Source: CAD feature listing. Evaluate the final solid. Frame: model axes, mm. A direction names the side the tool comes from. Give positions to 0.01 mm unless a question says otherwise; leave off trailing zeros. Write each loop counter-clockwise with the first axis right and the second up, starting at its lowest first coordinate (ties: lowest second). Pieces come first, ordered by that corner, then holes. Notation, with made-up numbers: M 33.25,37 L 39.25,37 A21 cw 39.25,72 Z; hole C 79.5,33 d4. An arc over 180 degrees is marked long. Return JSON: item names as keys, results as strings.
Autodesk Inventor part; units mm, degrees
ref_plane "YZ Plane" through (0, 0, 0) normal (1, 0, 0) x (0, 1, 0)
ref_plane "XZ Plane" through (0, 0, 0) normal (0, 1, 0) x (-1, 0, 0)
ref_plane "XY Plane" through (0, 0, 0) normal (0, 0, 1) x (1, 0, 0)
sketch "Sketch1" plane through (0, 0, 0) normal (0, 0, 1) x (1, 0, 0)
  line L0 (-0.7879, 4.5) -> (3.5032, 2.9324)
  line L1 (3.5032, 2.9324) -> (4.2911, -1.5676)
  line L2 (4.2911, -1.5676) -> (0.7879, -4.5)
  line L3 (0.7879, -4.5) -> (-3.5032, -2.9324)
  line L4 (-3.5032, -2.9324) -> (-4.2911, 1.5676)
  line L5 (-4.2911, 1.5676) -> (-0.7879, 4.5)
  point P0 (0, 0)
  point P1 (0, 0)
  dimension "d0" = 9
extrude "Extrusion1" add sketch "Sketch1" along normal blind 3
sketch "Sketch2" plane through (0, 0, 3) normal (0, 0, 1) x (1, 0, 0)
  circle A0 centre (0, 0) radius 3
  dimension "d3" = 6
extrude "Extrusion2" add sketch "Sketch2" along normal blind 1
sketch "Sketch3" plane through (0, 0, 4) normal (0, 0, 1) x (1, 0, 0)
  line L0 (-0.7879, 4.5) -> (-4.2911, 1.5676)
  line L1 (-0.7879, 4.5) -> (3.5032, 2.9324)
  line L2 (3.5032, 2.9324) -> (4.2911, -1.5676)
  line L3 (4.2911, -1.5676) -> (0.7879, -4.5)
  line L4 (0.7879, -4.5) -> (-3.5032, -2.9324)
  line L5 (-3.5032, -2.9324) -> (-4.2911, 1.5676)
  line L6 (-4.2911, 1.5676) -> (-0.7879, 4.5)
  point P0 (0, 0)
  point P1 (0, 0)
extrude "Extrusion3" add sketch "Sketch3" along normal blind 3
sketch "Sketch4" plane through (0, 0, 7) normal (0, 0, 1) x (1, 0, 0)
  circle A0 centre (0, 0) radius 3
  dimension "d8" = 6
extrude "Extrusion4" add sketch "Sketch4" along normal blind 22
thread "Thread1"
properties part number "HUDOSN-1-54B"
1) Set-up query: faces 4 (the face through (-3, 0, 18)), 5 (the face through (-3, -0.1, 3.5)), 6 (the face through (-1.328, -3.727, 1.479)). Return all of +Z, -Z, +X, -X, +Y, -Y with unobstructed straight access to the full face (end or side cutting, diameter ignored); none if empty.
Numbers:
{"face 4": "+Z", "face 5": "none", "face 6": "+Z, -Z, -X, -Y"}
2) Cut plane A-A, the plane y = 3.75. Return the cut outline in (x, z), then the cut area to 3 significant figures.
Numbers:
{"outline": "M -1.68,0 L 1.27,0 L 1.27,3 L -1.68,3 Z; M -1.68,4 L 1.27,4 L 1.27,7 L -1.68,7 Z", "area": "17.7 mm²"}
3) Contact query for flat-ended pins moving along their axis: pin 1 Ø5 at (x, z) = (1, 23.5) entering from -Y; pin 2 Ø1 at (y, z) = (1.5, 16) entering from -X; pin 3 Ø1.5 at (y, z) = (3, 16.5) entering from +X. Output: stop coordinate, or through.
Numbers:
{"pin 1": "stops at y = -3", "pin 2": "stops at x = -2.83", "pin 3": "stops at x = 1.98"}
4) Cut plane C-C, the plane z = 11.25. Return the cut outline in (x, y), then the cut area to 3 significant figures.
Numbers:
{"outline": "C 0,0 d6", "area": "28.3 mm²"}
5) Cut plane B-B, the plane x = -0.5. Return the cut outline in (y, z).
Numbers:
{"outline": "M -4.03,0 L 4.39,0 L 4.39,3 L 2.96,3 L 2.96,4 L 4.39,4 L 4.39,7 L 2.96,7 L 2.96,29 L -2.96,29 L -2.96,7 L -4.03,7 L -4.03,4 L -2.96,4 L -2.96,3 L -4.03,3 Z"}
6) Draft query along Z for faces 1 (the face through (-1, -3, 7)), 2 (the face through (-1, -3, 3)), 3 (the face through (2.564, -3.013, 1.479)). Return one class per face: released by +Z, released by -Z, zero draft, split by the parting line, or undercut.
Numbers:
{"face 1": "released by +Z", "face 2": "undercut", "face 3": "zero draft"}
7) Line query: line 1 (Z direction, x = 3.75, y = -1.75); line 2 (Y direction, x = 0, z = 26.75); line 3 (X direction, y = 1.75, z = 24). Output: solid intervals per line, ascending. Write a range as [from, to].
Numbers:
{"line 1": "z = [0, 3], [4, 7]", "line 2": "y = [-3, 3]", "line 3": "x = [-2.44, 2.44]"}
8) Cut plane D-D, the plane y = 0. Return the cut outline in (x, z), then the cut area to 3 significant figures.
Numbers:
{"outline": "M -4.02,0 L 4.02,0 L 4.02,3 L 3,3 L 3,4 L 4.02,4 L 4.02,7 L 3,7 L 3,29 L -3,29 L -3,7 L -4.02,7 L -4.02,4 L -3,4 L -3,3 L -4.02,3 Z", "area": "186 mm²"}
